```python
from build123d import *

# Parameters (mm, degrees)
F1_DEPTH = 3.81
F2_R     = 1.27
F3_DEPTH = 25.4
F4_R     = 1.27
F5_DEPTH = 9.4996


with BuildPart() as f1:
    # F0 (on Right) → F1 (new body)
    with BuildSketch(Plane.YZ):
        with BuildLine():
            Line((0, 4.382191), (0, 0))
            Line((0, 0), (2.54, 0))
            Line((2.54, 0), (2.54, 4.228206))
            ThreePointArc((2.54, 4.228206), (2.252063, 6.118681), (1.414363, 7.837711))
            ThreePointArc((1.414363, 7.837711), (-2.381643, 21.423937), (3.005292, 34.461426))
            ThreePointArc((3.005292, 34.461426), (4.186454, 36.41869), (4.597952, 38.667399))
            Line((4.597952, 38.667399), (4.597952, 43.971926))
            Line((4.597952, 43.971926), (2.54, 43.9214))
            Line((2.54, 43.9214), (2.54, 40.08054))
            ThreePointArc((2.54, 40.08054), (2.145807, 37.878073), (1.01217, 35.949054))
            ThreePointArc((1.01217, 35.949054), (-4.635087, 22.199709), (-0.991445, 7.7893))
            ThreePointArc((-0.991445, 7.7893), (-0.252897, 6.156406), (0, 4.382191))
        make_face()
    extrude(amount=F1_DEPTH)

    # F2 (on face) → F3 (cut)
    with BuildSketch(Plane.XZ.offset(-2.54)):
        with Locations((1.905, 42.00097)):
            Circle(F2_R)
    extrude(amount=-F3_DEPTH, mode=Mode.SUBTRACT)

    # F4 (on face) → F5 (cut)
    with BuildSketch(Plane.XZ):
        with Locations((1.905, 2.191095)):
            Circle(F4_R)
    extrude(amount=-F5_DEPTH, mode=Mode.SUBTRACT)


solid = f1.part
```
Build history of the part. All positions in model axes, mm. A direction names the side the tool comes from. Round coordinates to 2 decimals unless told otherwise and drop trailing zeros. Write each loop counter-clockwise with the first axis right and the second up, starting at its lowest first coordinate (ties: lowest second). Pieces come first, ordered by that corner, then holes. Notation, with made-up numbers: (38.5, -40) -> (87.5, -40) arc R37 cw to (87.5, -2) -> close; hole circle Ø4 at (-18, 34). An arc over 180 degrees is marked (long way). Put each result on its own line as item: value.
Item 1: Slice it at B-B, the plane x = 2.8. Give the cut face in (y, z).
Here are the results:
outline: (-0.99, 7.79) arc R6.35 cw to (0, 4.38) -> (0, 3.09) -> (2.54, 3.09) -> (2.54, 4.23) arc R6.35 ccw to (1.41, 7.84) arc R21.63 cw to (3.01, 34.46) arc R6.35 ccw to (4.6, 38.67) -> (4.6, 41.1) -> (2.54, 41.1) -> (2.54, 40.08) arc R6.35 cw to (1.01, 35.95) arc R23.72 ccw to start; (0, 0) -> (2.54, 0) -> (2.54, 1.29) -> (0, 1.29) -> close; (2.54, 42.9) -> (4.6, 42.9) -> (4.6, 43.97) -> (2.54, 43.92) -> close
Item 2: Slice it at D-D, the plane y = 4. Give the cut face in (x, z) (3 decimals).
Here are the results:
outline: (0, 35.977) -> (3.81, 35.977) -> (3.81, 43.957) -> (0, 43.957) -> close; hole circle Ø2.54 at (1.905, 42.001)
Item 3: Slice it at A-A, the plane y = 0.5. Give the cut face in (x, z) (3 decimals), plus the area to 3 significant figures.
Here are the results:
outline: (0, 0) -> (3.81, 0) -> (3.81, 9.28) -> (0, 9.28) -> close; (0, 30.988) -> (3.81, 30.988) -> (3.81, 35.33) -> (0, 35.33) -> close; hole circle Ø2.54 at (1.905, 2.191)
area: 46.8 mm^2
Item 4: Slice it at C-C, the plane y = -1.5. Give the cut face in (x, z), plus the area to 3 significant figures.
Here are the results:
outline: (0, 8.63) -> (3.81, 8.63) -> (3.81, 13.89) -> (0, 13.89) -> close; (0, 26.38) -> (3.81, 26.38) -> (3.81, 32.41) -> (0, 32.41) -> close
area: 43.0 mm^2
Item 5: Two-plate mould, pull along X, no slides. Class faces 4 (the face through (1.63, 1.25, 0.95)), 5 (the face through (1.88, -4.62, 22.41)), 6 (the face through (3.81, -2.5, 23.7)): pulls with the +X half, pulls with the -X half, needs draft (parallel to the pull), parting line crosses it, or undercut.
Here are the results:
face 4: undercut
face 5: needs draft
face 6: pulls with the +X half
Item 6: Tool access for faces 1 (the face through (1.88, 2.26, 6.09)), 2 (the face through (1, 0, 1)), 3 (the face through (1, 2.54, 1)): list every direction of +Z, -Z, +X, -X, +Y, -Y with a clear straight run to the whole face (end or side of a thin tool).
Here are the results:
face 1: +X, -X, +Y
face 2: -Z, +X, -X, -Y
face 3: -Z, +X, -X, +Y
Item 7: Wall check: probe 1 along Z at (x, y) = (1.85, 1); probe 2 along Z at (x, y) = (2.8, 1.5); probe 3 along Y at (x, z) = (3.45, 41.5). Give the ranges that are in metal, low to high. Write a range as from..to.
Here are the results:
probe 1: z = 0..0.92, 3.46..8.46, 31.81..35.93
probe 2: z = 0..1.29, 3.09..7.71, 32.55..36.6
probe 3: y = 2.54..4.6
Item 8: Flat gauge pins, fed straight in: P1, Ø2, axis at x = 2, z = 36.5, coming from the +Y side; P2, Ø2, axis at x = 1.9, z = 42, coming from the +Y side; P3, Ø1.9, axis at x = 1, z = 1.5, coming from the +Y side; P4, Ø1, axis at x = 3, z = 19.5, coming from the -Y side. Where does each tip first touch, or does it go through?
Here are the results:
P1: stops at y = 4.49
P2: passes through
P3: stops at y = 2.54
P4: stops at y = -4.69
